Could you check a few things on this model? Use its own coordinates, in mm. Face numbers are marked on the shaded views. A direction names the side the tool comes from. Round coordinates to 2 decimals unless told otherwise and drop trailing zeros. Order: outer loops, then holes, each group sorted by start corner. A loop starts at its lowest first (then second) coordinate and runs counter-clockwise, first axis right, second up. Notation, with made-up numbers: (70, 41.5) -> (99, 41.5) arc R17 ccw to (99, 69.5) -> close; hole circle Ø7 at (26.25, -39.5). An arc over 180 degrees is marked (long way). One line per question, with ' | ' between items.
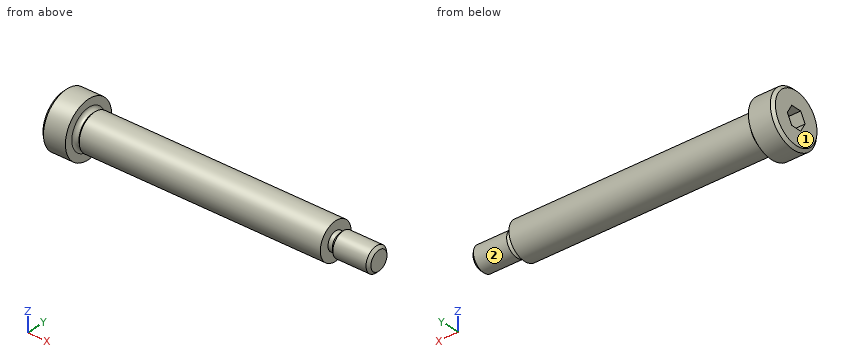
```python
from build123d import *

# Parameters (mm, degrees)
ENL_V_MAT_EXTRU_1_DEPTH = 2


with BuildPart() as part:
    # Esquisse1 → Révolution1 (revolve)
    with BuildSketch(Plane.XY, mode=Mode.PRIVATE) as r_volution1_sk:
        with BuildLine():
            Line((-1.133974596, 0), (-2, 1.5))
            Line((-2, 1.5), (-4, 1.5))
            Line((-4, 1.5), (-4, 4.05))
            Line((-4, 4.05), (-3.55, 4.5))
            Line((-3.55, 4.5), (0, 4.5))
            Line((0, 4.5), (0, 3.25))
            ThreePointArc((0, 3.25), (0.219643047, 2.809091151), (0.7, 2.7))
            Line((0.7, 2.7), (1, 3))
            Line((1, 3), (40, 3))
            Line((40, 3), (40, 1.5))
            Line((40, 1.5), (40.7, 1.5))
            Line((40.7, 1.5), (41.2, 2))
            Line((41.2, 2), (46.5705, 2))
            Line((46.5705, 2), (47, 1.5705))
            Line((47, 1.5705), (47, 0))
            Line((47, 0), (-1.133974596, 0))
        make_face()
    revolve(r_volution1_sk.sketch.rotate(Axis((47, 0, 0), (-1, 0, 0)), 270), axis=Axis((47, 0, 0), (-1, 0, 0)))

    # Esquisse2 → Enlèv. mat.-Extru.1 (cut)
    with BuildSketch(Plane(origin=(-4, 0, 0), x_dir=(0, 0, -1), z_dir=(1, 0, 0))):
        Polygon((-1.5, 0.866025404), (-1.5, -0.866025404), (0, -1.732050808), (1.5, -0.866025404), (1.5, 0.866025404), (0, 1.732050808), align=None)
    extrude(amount=ENL_V_MAT_EXTRU_1_DEPTH, mode=Mode.SUBTRACT)


solid = part.part
```
1. I'm going to push flat-ended pins straight in: pin 1 (4 mm diameter, centred on y = 2.5, z = 3.5, fed in from +X); pin 2 (1.5 mm diameter, centred on x = 12, y = -3, fed in from -Z). Where does each tip first touch, or does it pass through?
From the geometry:
pin 1: stops at x = 40 | pin 2: stops at z = -1.98
2. I need wall thicknesses on probe 1 along X at (y, z) = (-0.5, 2); probe 2 along X at (y, z) = (2, -3); probe 3 along Y at (x, z) = (26, 0.25). Which ranges of each line are inside material? Lowest first, please.
From the geometry:
probe 1: x = -4 to 40 | probe 2: x = -4 to 0 | probe 3: y = -2.99 to 2.99
3. I want a section at A-A on x = 18.5. List the corners of the cut face in (y, z) for me.
From the geometry:
outline: circle Ø6 at (0, 0)
4. On a 3-axis mill with a long thin cutter (end or side, diameter ignored), from which of +Z, -Z, +X, -X, +Y, -Y can I reach the whole of each face in a straight line? I mean the marked faces 1 and 2. Say none if no direction works.
From the geometry:
face 1: +Z, -Z, -X, +Y, -Y | face 2: +X
